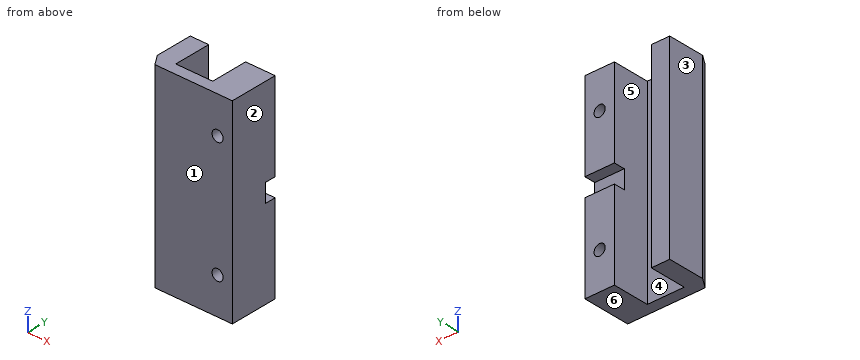
Autodesk Inventor part; units mm, degrees
ref_plane "YZ Plane" through (0, 0, 0) normal (1, 0, 0) x (0, 1, 0)
ref_plane "XZ Plane" through (0, 0, 0) normal (0, 1, 0) x (-1, 0, 0)
ref_plane "XY Plane" through (0, 0, 0) normal (0, 0, 1) x (1, 0, 0)
sketch "Boceto1" plane through (0, 0, 0) normal (0, 1, 0) x (-1, 0, 0)
  line L0 (9.0356, 45.002) -> (-13.9644, 45.002)
  line L1 (-13.9644, 45.002) -> (-13.9644, -7.998)
  line L2 (-13.9644, -7.998) -> (9.0356, -7.998)
  line L3 (9.0356, -7.998) -> (9.0356, 45.002)
  point P0 (0, 0)
  dimension "d0" = 23
  dimension "d1" = 53
extrude "Extrusión1" add sketch "Boceto1" along normal blind 3
sketch "Boceto2" plane through (0, 3, 0) normal (0, 1, 0) x (1, 0, 0)
  line L0 (-9.0356, -45.002) -> (13.9644, -45.002)
  line L1 (13.9644, -45.002) -> (13.9644, 7.998)
  line L2 (5.9644, -45.002) -> (13.9644, -45.002)
  line L3 (13.9644, -45.002) -> (13.9644, 7.998)
  line L4 (13.9644, 7.998) -> (5.9644, 7.998)
  line L5 (5.9644, 7.998) -> (5.9644, -45.002)
  point P0 (0, 0)
  dimension "d4" = 8
extrude "Extrusión2" add sketch "Boceto2" along normal blind 10
sketch "Boceto3" plane through (0, 13, 0) normal (0, 1, 0) x (1, 0, 0)
  line L0 (5.9644, 7.998) -> (5.9644, -45.002)
  line L1 (5.9644, -21.002) -> (13.9831, -21.002)
  line L2 (13.9831, -21.002) -> (13.9831, -16.002)
  line L3 (13.9831, -16.002) -> (5.9644, -16.002)
  line L4 (5.9644, -16.002) -> (5.9644, -21.002)
  line L5 (13.9644, 7.998) -> (5.9644, 7.998)
  line L6 (5.9644, -45.002) -> (13.9644, -45.002)
  point P0 (0, 0)
  dimension "d7" = 24
  dimension "d8" = 5
  dimension "d9" = 24
extrude "Extrusión3" cut sketch "Boceto3" against normal blind 3
sketch "Boceto4" plane through (0, 13, 0) normal (0, 1, 0) x (1, 0, 0)
  circle A0 centre (9.9644, -2.002) radius 1.5
  line L0 (13.9644, 7.998) -> (5.9644, 7.998)
  line L1 (13.9644, -16.002) -> (13.9644, 7.998)
  line L2 (13.9644, -45.002) -> (13.9644, 7.998)
  line L3 (13.9644, -18.502) -> (5.9644, -18.502)
  circle A1 centre (9.9644, -35.002) radius 1.5
  point P0 (0, 0)
  dimension "d12" = 3
  dimension "d13" = 10
  dimension "d14" = 4
extrude "Extrusión4" cut sketch "Boceto4" against normal blind 14.75
sketch "Boceto5" plane through (0, 3, 0) normal (0, 1, 0) x (1, 0, 0)
  line L0 (-9.0356, -45.002) -> (-4.0356, -45.002)
  line L1 (-4.0356, -45.002) -> (-4.0356, 7.998)
  line L2 (-4.0356, 7.998) -> (-9.0356, 7.998)
  line L3 (-9.0356, 7.998) -> (-9.0356, -45.002)
  point P0 (0, 0)
  dimension "d17" = 5
extrude "Extrusión5" add sketch "Boceto5" along normal blind 10
sketch "Boceto7" plane through (13.9644, 0, -7.998) normal (0, 0, -1) x (-1, 0, 0)
  line L0 (23, 0) -> (21, 0)
  line L1 (23, 0) -> (0, 0)
  line L2 (23, 0) -> (23, 3)
  line L3 (21, 0) -> (23, 3)
  point P0 (13.9644, 0)
  dimension "d24" = 2
  dimension "d25" = 3
extrude "Extrusión7" cut sketch "Boceto7" against normal blind 55.5
sketch "Boceto8" plane through (13.9644, 0, 45.002) normal (1, 0, 0) x (0, 0, -1)
  point P0 (45.002, 0)
equation "\"Radio_pliegue\" = Grosor"
equation "\"Anchura_desahogo_plegado\" = Grosor"
equation "\"Profundidad_desahogo_plegado\" = 0.5 * Grosor"
equation "\"Tamaño_destalonado\" = 4 * Grosor"
equation "\"Remanente_mínimo\" = 2 * Grosor"
equation "\"Radiodetransición\" = Radio_pliegue"
equation "\"Tamaño_de_radio_de_Jacobi\" = Radio_pliegue"
equation "\"TamañoSeparación\" = Grosor"
properties part number "PiezaAtras"
CAD build for the part. Positions are in the model's coordinates, mm. Face numbers are marked on the shaded views. A direction names the side the tool comes from. Coordinates: 2 decimals unless noted, no trailing zeros. Write each loop counter-clockwise with the first axis right and the second up, starting at its lowest first coordinate (ties: lowest second). Pieces come first, ordered by that corner, then holes.
(1) Cut at D-D, the plane z = 24.5. List the corners of the cut face in (x, y).
(2) Drill centre lines: probe 1 along X at (y, z) = (7.5, 30.5); probe 2 along X at (y, z) = (10, 3); probe 3 along Z at (x, y) = (10.75, 10.5). Where is each one in solid material? Low to high.
(3) Two-plate mould, pull along X, no slides. Class the marked faces 1, 2, 3 and 4: +X half, -X half, draft (parallel to the pull), parting line (faces both ways), or undercut.
(4) Flat gauge pin, fed straight in: pin 1 (2.5 mm diameter, centred on x = 10.5, z = 19, fed in from +Y). Where does the tip first touch, or does it go through?
(5) 3-axis set-ups, long thin cutter, end or side, ignore diameter. For the marked faces 5 and 6: which of +Z, -Z, +X, -X, +Y, -Y reach the whole face in a straight line?
(6) Cut at B-B, the plane y = 12. List the corners of the cut face in (x, z), and give its area (3 significant figures).
(7) Cut at A-A, the plane y = 5. List the corners of the cut face in (x, z).
(8) Cut at C-C, the plane x = 10.75. List the corners of the cut face in (y, z), and give its area (3 significant figures).
Geometry says:
1. outline: (-9.04, 3) - (-7.04, 0) - (13.96, 0) - (13.96, 13) - (5.96, 13) - (5.96, 3) - (-4.04, 3) - (-4.04, 13) - (-9.04, 13) - close
2. probe 1: x = -9.04 to -4.04, 5.96 to 13.96
2. probe 2: x = -9.04 to -4.04, 5.96 to 8.84, 11.08 to 13.96
2. probe 3: z = -8 to 0.72, 3.28 to 16, 21 to 33.72, 36.28 to 45
3. face 1: draft
3. face 2: +X half
3. face 3: -X half
3. face 4: undercut
4. pin 1: stops at y = 10
5. face 5: +Z, -Z, +Y
5. face 6: -Z, +X, -X, +Y, -Y
6. outline: (-9.04, -8) - (-4.04, -8) - (-4.04, 45) - (-9.04, 45) - close; (5.96, -8) - (13.96, -8) - (13.96, 16) - (5.96, 16) - close; (5.96, 21) - (13.96, 21) - (13.96, 45) - (5.96, 45) - close; hole circle Ø3 at (9.96, 2); hole circle Ø3 at (9.96, 35)
6. area: 635 mm2
7. outline: (-9.04, -8) - (-4.04, -8) - (-4.04, 45) - (-9.04, 45) - close; (5.96, -8) - (13.96, -8) - (13.96, 45) - (5.96, 45) - close; hole circle Ø3 at (9.96, 2); hole circle Ø3 at (9.96, 35)
8. outline: (0, -8) - (13, -8) - (13, 0.72) - (0, 0.72) - close; (0, 3.28) - (13, 3.28) - (13, 16) - (10, 16) - (10, 21) - (13, 21) - (13, 33.72) - (0, 33.72) - close; (0, 36.28) - (13, 36.28) - (13, 45) - (0, 45) - close
8. area: 608 mm2
